```python
from build123d import *

# Parameters (mm, degrees)
EXTRUDE_1_DEPTH     = 1.6
CUT_EXTRUDE_1_DEPTH = 10
SKETCH_3_R          = 1.6
CUT_EXTRUDE_2_DEPTH = 94.525061209
CUT_EXTRUDE_3_DEPTH = 5


with BuildPart() as part:
    # 草图1 → 凸台-拉伸1 (new body)
    with BuildSketch(Plane(origin=(0, 0, 0), x_dir=(1, 0, 0), z_dir=(0, 1, 0))):
        with BuildLine():
            Line((7.841679065, 0), (77.841679065, 0))
            ThreePointArc((77.841679065, 0), (79.962999409, 0.878679656), (80.841679065, 3))
            Line((80.841679065, 3), (80.841679065, 7))
            ThreePointArc((80.841679065, 7), (79.962999409, 9.121320344), (77.841679065, 10))
            Line((77.841679065, 10), (66.341679065, 10))
            ThreePointArc((66.341679065, 10), (64.220358721, 10.878679656), (63.341679065, 13))
            Line((63.341679065, 13), (63.341679065, 44))
            ThreePointArc((63.341679065, 44), (62.462999409, 46.121320344), (60.341679065, 47))
            Line((60.341679065, 47), (25.341679065, 47))
            ThreePointArc((25.341679065, 47), (23.220358721, 46.121320344), (22.341679065, 44))
            Line((22.341679065, 44), (22.341679065, 13))
            ThreePointArc((22.341679065, 13), (21.462999409, 10.878679656), (19.341679065, 10))
            Line((19.341679065, 10), (7.841679065, 10))
            ThreePointArc((7.841679065, 10), (5.720358721, 9.121320344), (4.841679065, 7))
            Line((4.841679065, 7), (4.841679065, 3))
            ThreePointArc((4.841679065, 3), (5.720358721, 0.878679656), (7.841679065, 0))
        make_face()
    extrude(amount=EXTRUDE_1_DEPTH)

    # 草图2 → 切除-拉伸1 (cut)
    with BuildSketch(Plane(origin=(0, 1.6, 0), x_dir=(1, 0, 0), z_dir=(0, 1, 0))):
        with BuildLine():
            Line((37.841679065, 1), (37.841679065, 4))
            ThreePointArc((37.841679065, 4), (38.134572284, 4.707106781), (38.841679065, 5))
            Line((38.841679065, 5), (46.841679065, 5))
            ThreePointArc((46.841679065, 5), (47.548785846, 4.707106781), (47.841679065, 4))
            Line((47.841679065, 4), (47.841679065, 1))
            ThreePointArc((47.841679065, 1), (48.134572284, 0.292893219), (48.841679065, 0))
            Line((48.841679065, 0), (36.841679065, 0))
            ThreePointArc((36.841679065, 0), (37.548785846, 0.292893219), (37.841679065, 1))
        make_face()
    extrude(amount=-CUT_EXTRUDE_1_DEPTH, mode=Mode.SUBTRACT)

    # 草图3 → 切除-拉伸2 (cut, through all)
    with BuildSketch(Plane(origin=(0, 1.6, 0), x_dir=(1, 0, 0), z_dir=(0, 1, 0))):
        with Locations(Location((7.841679065, 7, 0), (0, 0, 270))):
            Circle(SKETCH_3_R)
        with Locations(Location((29.841679065, 3, 0), (0, 0, 270))):
            Circle(SKETCH_3_R)
        with Locations(Location((25.341679065, 44, 0), (0, 0, 270))):
            Circle(SKETCH_3_R)
        with Locations(Location((60.341679065, 44, 0), (0, 0, 90))):
            Circle(SKETCH_3_R)
        with Locations(Location((55.841679065, 3, 0), (0, 0, 90))):
            Circle(SKETCH_3_R)
        with Locations(Location((77.841679065, 7, 0), (0, 0, 90))):
            Circle(SKETCH_3_R)
    extrude(amount=-CUT_EXTRUDE_2_DEPTH, mode=Mode.SUBTRACT)

    # 草图4 → 切除-拉伸3 (cut)
    with BuildSketch(Plane(origin=(0, 1.6, 0), x_dir=(1, 0, 0), z_dir=(0, 1, 0))):
        with BuildLine():
            Line((46.841679065, 45), (46.841679065, 46))
            ThreePointArc((46.841679065, 46), (47.134572284, 46.707106781), (47.841679065, 47))
            Line((47.841679065, 47), (37.841679065, 47))
            ThreePointArc((37.841679065, 47), (38.548785846, 46.707106781), (38.841679065, 46))
            Line((38.841679065, 46), (38.841679065, 45))
            ThreePointArc((38.841679065, 45), (42.841679065, 41), (46.841679065, 45))
        make_face()
    extrude(amount=-CUT_EXTRUDE_3_DEPTH, mode=Mode.SUBTRACT)


solid = part.part
```
The listing builds one solid part. Answer for the finished solid, in the listing's coordinates (mm). A direction names the side the tool comes from. Coordinates: 2 decimals unless noted, no trailing zeros. Write each loop counter-clockwise with the first axis right and the second up, starting at its lowest first coordinate (ties: lowest second). Pieces come first, ordered by that corner, then holes.
Q1. Section A-A, the plane x = 24.5 is taken. Write down the section's boundary in (y, z), then the cut area to 3 significant figures.
Returned:
outline: (0, -46.88) - (1.6, -46.88) - (1.6, -45.36) - (0, -45.36) - close; (0, -42.64) - (1.6, -42.64) - (1.6, 0) - (0, 0) - close
area: 70.7 mm2
Q2. Section B-B, the plane z = -29 is taken. Write down the section's boundary in (x, y).
Returned:
outline: (22.34, 0) - (63.34, 0) - (63.34, 1.6) - (22.34, 1.6) - close
Q3. Section D-D, the plane y = 1.25 is taken. Give the number of separate pieces and of enclosed holes in the cut face, then the cut area to 3 significant figures.
Returned:
separate pieces: 1
enclosed holes: 6
area: 2,130 mm2
Q4. Find the intervals of material crossed by line 1 along X through (y, z) = (0.5, -7); line 2 along X through (y, z) = (0.75, -44); line 3 along Z through (x, y) = (78, 0.25), in increasing order.
Returned:
line 1: x = 4.84 to 6.24, 9.44 to 76.24, 79.44 to 80.84
line 2: x = 22.34 to 23.74, 26.94 to 38.97, 46.71 to 58.74, 61.94 to 63.34
line 3: z = -10 to -8.59, -5.41 to 0
Q5. Section C-C, the plane x = 75 is taken. Write down the section's boundary in (y, z).
Returned:
outline: (0, -10) - (1.6, -10) - (1.6, 0) - (0, 0) - close
Q6. Which of the six approach directions +Z, -Z, +X, -X, +Y, -Y give full straight-line access (tool end or side, diameter ignored) to faces 1 (the flat face through (47.842, 1, -3)), 2 (the cylindrical face through (5.7, 0.8, -0.9)), 3 (the flat face through (14, 1, -10)), 4 (the flat face through (72, 1, -10))?
Returned:
face 1: +Z, +Y, -Y
face 2: +Z, -X, +Y, -Y
face 3: -Z, -X, +Y, -Y
face 4: -Z, +X, +Y, -Y
Q7. The mould has two halves that part along X. Classify faces 5 (the cylindrical face through (31.428, 0.811, -3.208)), 6 (the flat face through (42, 1.6, -19)), 7 (the cylindrical face through (79.986, 0.789, -9.098)), 8 (the flat face through (37.842, 1, -2)): released by +X, released by -X, zero draft, split by the parting line, or undercut.
Returned:
face 5: undercut
face 6: zero draft
face 7: released by +X
face 8: undercut
Q8. Given P1, Ø0.8, axis at x = 73.5, y = 1, coming from the -Z side; P2, Ø0.5, axis at y = 0.5, z = -21, coming from the -X side, each flat-ended and moving along its own axis, determine where each tip first touches the part or whether it passes through.
Returned:
P1: stops at z = -10
P2: stops at x = 22.34
